Here's how the part is built. I have some questions about the finished solid (model axes, mm). Face numbers are marked on the shaded views. A direction names the side the tool comes from. Round coordinates to 2 decimals unless told otherwise and drop trailing zeros. Order: outer loops, then holes, each group sorted by start corner. A loop starts at its lowest first (then second) coordinate and runs counter-clockwise, first axis right, second up. Notation, with made-up numbers: (65, -15) -> (73, -15) arc R11 ccw to (73, 1) -> close; hole circle Ø10 at (79.25, -35.5). An arc over 180 degrees is marked (long way). Answer in a Markdown table with one row per item.
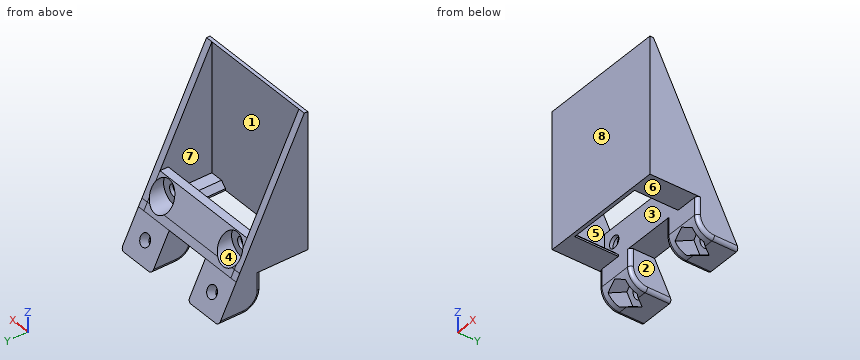
```python
from build123d import *

# Parameters (mm, degrees)
BOSS_EXTRUDE1_DEPTH             = 16.25
CUT_EXTRUDE7_DEPTH              = 47.531565279
CUT_EXTRUDE7_DEPTH_BACK         = 47.531565279
SKETCH2_W                       = 22.3
SKETCH2_H                       = 12.5
CUT_EXTRUDE1_DEPTH              = 26.461981463
BOSS_EXTRUDE2_DEPTH             = 2
BOSS_EXTRUDE4_REACH             = 49.267
BOSS_EXTRUDE4_DIRECTION_2_REACH = 49.267
SKETCH12_R                      = 1.75
CUT_EXTRUDE8_DEPTH              = 45.835104186
CUT_EXTRUDE10_START             = -1
SKETCH14_R                      = 4
CUT_EXTRUDE10_DEPTH             = 44.835104186
SKETCH15_W                      = 36.5
SKETCH15_H                      = 38.998385445
BOSS_EXTRUDE5_DEPTH             = 1
BOSS_EXTRUDE6_DEPTH             = 36.5
SKETCH18_W                      = 13.5
SKETCH18_H                      = 10
CUT_EXTRUDE12_DEPTH             = 46.124124006
SKETCH21_R                      = 1.75
CUT_EXTRUDE15_DEPTH             = 40.773623022
CUT_EXTRUDE16_START             = -3
CUT_EXTRUDE16_DEPTH             = 37.773623022
CHAMFER1_SIZE                   = 1.5
FILLET1_R                       = 5
FILLET2_R                       = 1


with BuildPart() as part:
    # Sketch1 → Boss-Extrude1 (new, symmetric)
    with BuildSketch(Plane(origin=(0, 0, 0), x_dir=(0, 0, -1), z_dir=(1, 0, 0))):
        Polygon((0, 19.5), (0, 0), (-38.998385445, 0), align=None)
    extrude(amount=BOSS_EXTRUDE1_DEPTH, both=True)

    # Sketch10 → Cut-Extrude7 (cut, two sides: drawn at the far end of the back side and taken through both)
    with BuildSketch(Plane(origin=(0, 0, 0), x_dir=(0, 0, -1), z_dir=(1, 0, 0)).offset(-CUT_EXTRUDE7_DEPTH_BACK)):
        Polygon((-2, 0), (-2, 18.499958599), (-38.998385445, 0), align=None)
    extrude(amount=CUT_EXTRUDE7_DEPTH + CUT_EXTRUDE7_DEPTH_BACK, mode=Mode.SUBTRACT)

    # Sketch2 → Cut-Extrude1 (cut, through all)
    with BuildSketch(Plane.XY):
        with Locations((0, 6.25)):
            Rectangle(SKETCH2_W, SKETCH2_H)
    extrude(amount=CUT_EXTRUDE1_DEPTH, mode=Mode.SUBTRACT)

    # Sketch6 → Boss-Extrude2 (add)
    with BuildSketch(Plane(origin=(-16.25, 0, 0), x_dir=(0, 0, -1), z_dir=(1, 0, 0))):
        Polygon((-2, 0), (-38.998385445, 0), (-2, 18.499958599), (0, 19.5), (0, 0), align=None)
    boss_extrude2 = extrude(amount=-BOSS_EXTRUDE2_DEPTH)

    # Mirror1: Boss-Extrude2 across plane
    add(boss_extrude2.mirror(Plane(origin=(0, 0, 0), x_dir=(0, 0, 1), z_dir=(1, 0, 0))))

    # Boss-Extrude4: up to this face of the body (flat: up to its plane)
    boss_extrude4_end = Plane(part.part.faces().sort_by_distance((16.25, 6.166652866, 14.332795148))[0])
    # Sketch11 → Boss-Extrude4 (add, up to the picked face)
    with BuildSketch(Plane(origin=(0, 0, 0), x_dir=(0, 0, -1), z_dir=(1, 0, 0)), mode=Mode.PRIVATE) as boss_extrude4_sk1:
        Polygon((-2, 18.499958599), (-9.25, 14.874808522), (-9.25, 12.5), (-2, 12.5), align=None)
    boss_extrude4_tool1 = split(extrude(boss_extrude4_sk1.sketch, amount=BOSS_EXTRUDE4_REACH, mode=Mode.PRIVATE), bisect_by=boss_extrude4_end, keep=Keep.BOTH, mode=Mode.PRIVATE)
    add(boss_extrude4_tool1.solids().sort_by(Axis((0, 14.724459, 5.101954), (1, 0, 0)))[0])

    # Boss-Extrude4 direction 2: up to this face of the body (flat: up to its plane)
    boss_extrude4_direction_2_end = Plane(part.part.faces().sort_by_distance((-16.25, 6.166652866, 14.332795148))[0])
    # Sketch11 → Boss-Extrude4 direction 2 (add, up to the picked face)
    with BuildSketch(Plane(origin=(0, 0, 0), x_dir=(0, 0, -1), z_dir=(1, 0, 0)), mode=Mode.PRIVATE) as boss_extrude4_direction_2_sk1:
        Polygon((-2, 18.499958599), (-9.25, 14.874808522), (-9.25, 12.5), (-2, 12.5), align=None)
    boss_extrude4_direction_2_tool1 = split(extrude(boss_extrude4_direction_2_sk1.sketch, amount=-BOSS_EXTRUDE4_DIRECTION_2_REACH, mode=Mode.PRIVATE), bisect_by=boss_extrude4_direction_2_end, keep=Keep.BOTH, mode=Mode.PRIVATE)
    add(boss_extrude4_direction_2_tool1.solids().sort_by(Axis((0, 14.724459, 5.101954), (-1, 0, 0)))[0])

    # Sketch12 → Cut-Extrude8 (cut, through all)
    with BuildSketch(Plane.XZ.offset(-12.5)):
        with Locations(Location((-12.7, 5, 0), (0, 0, 270))):
            Circle(SKETCH12_R)
        with Locations(Location((12.7, 5, 0), (0, 0, 90))):
            Circle(SKETCH12_R)
    extrude(amount=-CUT_EXTRUDE8_DEPTH, mode=Mode.SUBTRACT)

    # Sketch14 → Cut-Extrude10 (cut, through all)
    with BuildSketch(Plane.XZ.offset(-12.5).offset(CUT_EXTRUDE10_START)):
        with Locations(Location((-12.7, 5, 0), (0, 0, 270))):
            Circle(SKETCH14_R)
        with Locations(Location((12.7, 5, 0), (0, 0, 270))):
            Circle(SKETCH14_R)
    extrude(amount=-CUT_EXTRUDE10_DEPTH, mode=Mode.SUBTRACT)

    # Sketch15 → Boss-Extrude5 (add)
    with BuildSketch(Plane.XZ):
        with Locations((0, 19.499192723)):
            Rectangle(SKETCH15_W, SKETCH15_H)
    extrude(amount=BOSS_EXTRUDE5_DEPTH)

    # Sketch17 → Boss-Extrude6 (add)
    with BuildSketch(Plane.ZY.offset(18.25)):
        Polygon((0, 19.5), (-10, 24.500207003), (-10, 12.5), (0, 12.5), align=None)
    extrude(amount=-BOSS_EXTRUDE6_DEPTH)

    # Sketch18 → Cut-Extrude12 (cut, through all)
    with BuildSketch(Plane.XZ.offset(-12.5)):
        with Locations((0, -5)):
            Rectangle(SKETCH18_W, SKETCH18_H)
    extrude(amount=-CUT_EXTRUDE12_DEPTH, mode=Mode.SUBTRACT)

    # Sketch21 → Cut-Extrude15 (cut, through all)
    with BuildSketch(Plane(origin=(0, 15.599741659, 7.800193749), x_dir=(1, 0, 0), z_dir=(0, 0.8944197849825609, 0.44722840722806245))):
        with Locations(Location((-12.5, 14.311170173, 0), (0, 0, 270))):
            Circle(SKETCH21_R)
        with Locations(Location((12.5, 14.311170173, 0), (0, 0, 172.6663404))):
            Circle(SKETCH21_R)
    extrude(amount=-CUT_EXTRUDE15_DEPTH, mode=Mode.SUBTRACT)

    # Sketch22 → Cut-Extrude16 (cut, through all)
    with BuildSketch(Plane(origin=(0, 15.599741659, 7.800193749), x_dir=(1, 0, 0), z_dir=(0, 0.8944197849825609, 0.44722840722806245)).offset(CUT_EXTRUDE16_START)):
        Polygon((12.5, 18.063946922), (9.25, 16.187558548), (9.25, 12.434781798), (12.5, 10.558393423), (15.75, 12.434781798), (15.75, 16.187558548), align=None)
        Polygon((-12.5, 18.063946922), (-15.75, 16.187558548), (-15.75, 12.434781798), (-12.5, 10.558393423), (-9.25, 12.434781798), (-9.25, 16.187558548), align=None)
    extrude(amount=-CUT_EXTRUDE16_DEPTH, mode=Mode.SUBTRACT)

    # Chamfer1
    chamfer1_edges = [part.edges().sort_by_distance(p)[0] for p in [
        (11.15, 6.25, 2),
        (-11.15, 6.25, 2),
    ]]
    chamfer(chamfer1_edges, length=CHAMFER1_SIZE)

    # Fillet1
    # the kernel refuses this fillet: 5 mm, written as the material it takes off along each edge
    with BuildSketch(Plane(origin=(-21.75, 12.5, -10), x_dir=(0, 0, 1), z_dir=(1, 0, 0)), Plane(origin=(3.25, 12.5, -10), x_dir=(0, 0, 1), z_dir=(1, 0, 0))) as fillet1_piece_1:
        with BuildLine():
            CenterArc((FILLET1_R, -FILLET1_R), FILLET1_R, 90, 90)
            Line((0, -FILLET1_R), (0, 0))
            Line((0, 0), (FILLET1_R, 0))
        make_face()
    extrude(amount=27.5, mode=Mode.SUBTRACT)

    # Fillet2
    fillet2_edges = [part.edges().sort_by_distance(p)[0] for p in [
        (-18.25, 21.000103501, -10),
        (18.25, 12.5, -2.5),
        (-6.75, 21.000103501, -10),
        (6.75, 21.000103501, -10),
        (-6.75, 12.5, -2.5),
        (-18.25, 12.5, -2.5),
        (-18.25, 13.964466094, -8.535533906),
        (6.75, 12.5, -2.5),
        (-6.75, 13.964466094, -8.535533906),
        (18.25, 21.000103501, -10),
        (6.75, 13.964466094, -8.535533906),
        (18.25, 13.964466094, -8.535533906),
    ]]
    fillet(fillet2_edges, radius=FILLET2_R)


solid = part.part
```
1. For the marked faces 1, 2, 3 and 4, which set-ups out of +Z, -Z, +X, -X, +Y, -Y let a thin tool reach every point of the face, with its end or its side?
Numbers:
| item | result |
|---|---|
| face 1 | +Z |
| face 2 | -Z, +Y, -Y |
| face 3 | none |
| face 4 | +Y |
2. Suppose I cut it at C-C on y = 9. Write out the boundary of the cut face in (x, z).
Numbers:
| item | result |
|---|---|
| outline | (-18.25, 0) -> (-11.15, 0) -> (-11.15, 0.5) -> (-12.65, 2) -> (-16.25, 2) -> (-16.25, 21) -> (-18.25, 21) -> close; (11.15, 0) -> (18.25, 0) -> (18.25, 21) -> (16.25, 21) -> (16.25, 2) -> (12.65, 2) -> (11.15, 0.5) -> close |
3. Suppose I cut it at A-A on x = 2. Write out the boundary of the cut face in (y, z).
Numbers:
| item | result |
|---|---|
| outline | (-1, 0) -> (0, 0) -> (0, 39) -> (-1, 39) -> close; (12.5, 0) -> (19.5, 0) -> (14.87, 9.25) -> (12.5, 9.25) -> close |
4. For pin 1 Ø5 at (x, z) = (1.5, 29) entering from +Y; pin 2 Ø3 at (x, y) = (-3.5, 12.5) entering from +Z; pin 3 Ø1.1 at (x, y) = (-14.5, 6.5) entering from +Z, each with a flat end and sliding along its axis, tell me the tip position at first contact or that it passes through.
Numbers:
| item | result |
|---|---|
| pin 1 | stops at y = 0 |
| pin 2 | stops at z = 9.25 |
| pin 3 | stops at z = 2 |
5. Suppose I cut it at D-D on z = 5. Write out the boundary of the cut face in (x, y).
Numbers:
| item | result |
|---|---|
| outline | (-18.25, -1) -> (18.25, -1) -> (18.25, 17) -> (16.7, 17) -> (16.7, 13.5) -> (14.45, 13.5) -> (14.45, 12.5) -> (16.25, 12.5) -> (16.25, 0) -> (-16.25, 0) -> (-16.25, 12.5) -> (-14.45, 12.5) -> (-14.45, 13.5) -> (-16.7, 13.5) -> (-16.7, 17) -> (-18.25, 17) -> close; (-10.95, 12.5) -> (10.95, 12.5) -> (10.95, 13.5) -> (8.7, 13.5) -> (8.7, 17) -> (-8.7, 17) -> (-8.7, 13.5) -> (-10.95, 13.5) -> close |
6. We'd pull the mould along Y, two halves only. Please class the marked faces 5, 6, 7 and 8: released by +Y, released by -Y, zero draft, split by the parting line, or undercut.
Numbers:
| item | result |
|---|---|
| face 5 | undercut |
| face 6 | zero draft |
| face 7 | undercut |
| face 8 | released by -Y |
7. Suppose I cut it at B-B on x = 13.5. Write out the boundary of the cut face in (y, z).
Numbers:
| item | result |
|---|---|
| outline | (-1, 0) -> (12.5, 0) -> (12.5, -5) arc R5 ccw to (12.63, -6.13) -> (17.9, -3.5) -> (18.67, -5.06) -> (21.36, -3.72) -> (18.96, 1.08) -> (13.5, 1.08) -> (13.5, 3.44) -> (12.5, 3.44) -> (12.5, 2) -> (0, 2) -> (0, 39) -> (-1, 39) -> close; (12.5, 6.56) -> (13.5, 6.56) -> (13.5, 8.92) -> (15.04, 8.92) -> (14.87, 9.25) -> (12.5, 9.25) -> close; (19.1, -10) -> (24.5, -10) -> (22.64, -6.28) -> (19.96, -7.63) -> (20.74, -9.18) -> close |
8. Please list where these lines run through material, in increasing order: line 1 along X through (y, z) = (13.1, 5); line 2 along X through (y, z) = (15.3, 5); line 3 along X through (y, z) = (19.5, -4).
Numbers:
| item | result |
|---|---|
| line 1 | x = -18.25 to -14.45, -10.95 to 10.95, 14.45 to 18.25 |
| line 2 | x = -18.25 to -16.7, -8.7 to 8.7, 16.7 to 18.25 |
| line 3 | x = -18.25 to -6.75, 6.75 to 18.25 |
